from build123d import *

# Parameters (mm, degrees)
BOSS_EXTRUDE1_DEPTH          = 9
SKETCH2_R                    = 2.766798225
SKETCH2_W                    = 278
SKETCH2_H                    = 187
CUT_EXTRUDE1_DEPTH           = 2
SKETCH4_W                    = 10
SKETCH4_H                    = 4
CUT_EXTRUDE2_DEPTH           = 2
CUT_EXTRUDE2_DRAFT           = -19
CUT_EXTRUDE2_PROFILE_2_DEPTH = 2
CUT_EXTRUDE2_PROFILE_2_DRAFT = -19


with BuildPart() as part:
    # Sketch1 → Boss-Extrude1 (new body)
    with BuildSketch(Plane(origin=(0, 0, 0), x_dir=(1, 0, 0), z_dir=(0, 1, 0))):
        with BuildLine():
            Line((-177.6, 71.8), (90.4, 71.8))
            ThreePointArc((90.4, 71.8), (97.471067812, 68.871067812), (100.4, 61.8))
            Line((100.4, 61.8), (100.4, -127.2))
            ThreePointArc((100.4, -127.2), (97.471067812, -134.271067812), (90.4, -137.2))
            Line((90.4, -137.2), (-177.6, -137.2))
            ThreePointArc((-177.6, -137.2), (-184.671067812, -134.271067812), (-187.6, -127.2))
            Line((-187.6, -127.2), (-187.6, 61.8))
            ThreePointArc((-187.6, 61.8), (-184.671067812, 68.871067812), (-177.6, 71.8))
        make_face()
    extrude(amount=BOSS_EXTRUDE1_DEPTH)

    # Sketch2 → Cut-Extrude1 (cut)
    with BuildSketch(Plane(origin=(0, 9, 0), x_dir=(1, 0, 0), z_dir=(0, 1, 0))):
        with Locations(Location((-43.280764326, 66.757707022, 0), (0, 0, 270))):
            Circle(SKETCH2_R)
        with Locations((-43.280764326, -32.742292978)):
            Rectangle(SKETCH2_W, SKETCH2_H)
    extrude(amount=-CUT_EXTRUDE1_DEPTH, mode=Mode.SUBTRACT)


with BuildPart() as cut_extrude2_tool:
    # Sketch4 → Cut-Extrude2 (with draft: the straight prism first)
    with BuildSketch(Plane.ZY.offset(187.6)):
        with Locations((-11.8, 4.5)):
            Rectangle(SKETCH4_W, SKETCH4_H)
    extrude(amount=-CUT_EXTRUDE2_DEPTH)
    # Cut-Extrude2: the draft: its side faces are tilted about the plane it starts from
    cut_extrude2_sides = [cut_extrude2_tool.faces().sort_by_distance(p)[0] for p in [
        (-186.6, 6.5, -11.8),
        (-186.6, 4.5, -16.8),
        (-186.6, 2.5, -11.8),
        (-186.6, 4.5, -6.8),
    ]]
    draft(cut_extrude2_sides, Plane.ZY.offset(187.6), CUT_EXTRUDE2_DRAFT)


with BuildPart() as part_1:
    add(part.part)

    # Cut-Extrude2: cut by cut_extrude2_tool
    add(cut_extrude2_tool.part, mode=Mode.SUBTRACT)


with BuildPart() as cut_extrude2_profile_2_tool:
    # Sketch4 → Cut-Extrude2 profile 2 (with draft: the straight prism first)
    with BuildSketch(Plane.ZY.offset(187.6)):
        with Locations((18.2, 4.5)):
            Rectangle(SKETCH4_W, SKETCH4_H)
    extrude(amount=-CUT_EXTRUDE2_PROFILE_2_DEPTH)
    # Cut-Extrude2 profile 2: the draft: its side faces are tilted about the plane it starts from
    cut_extrude2_profile_2_sides = [cut_extrude2_profile_2_tool.faces().sort_by_distance(p)[0] for p in [
        (-186.6, 2.5, 18.2),
        (-186.6, 4.5, 23.2),
        (-186.6, 6.5, 18.2),
        (-186.6, 4.5, 13.2),
    ]]
    draft(cut_extrude2_profile_2_sides, Plane.ZY.offset(187.6), CUT_EXTRUDE2_PROFILE_2_DRAFT)


with BuildPart() as part_2:
    add(part_1.part)

    # Cut-Extrude2 profile 2: cut by cut_extrude2_profile_2_tool
    add(cut_extrude2_profile_2_tool.part, mode=Mode.SUBTRACT)


solid = part_2.part
Here's how the part is built. I have some questions about the finished solid (model axes, mm). A direction names the side the tool comes from. Round coordinates to 2 decimals unless told otherwise and drop trailing zeros. Write each loop counter-clockwise with the first axis right and the second up, starting at its lowest first coordinate (ties: lowest second). Pieces come first, ordered by that corner, then holes.
1. Will these pins go through, and if not, where does the flat tip stop? pin 1 Ø8 at (x, z) = (19.5, 106) entering from +Y; pin 2 Ø0.8 at (y, z) = (4, -13.5) entering from -X.
2. Suppose I cut it at B-B (x = -73.5). List the corners of the cut face in (y, z) for me, and give its area (3 significant figures).
3. I need wall thicknesses on L1, parallel to Z at x = 44.5, y = 8; L2, parallel to X at y = 8, z = 68; L3, parallel to Y at x = 14.5, z = 117. Which ranges of each line are inside material? Lowest first, please.
4. If we mould it in two halves opening along X, with no side actions, what happens to faces 1 (the flat face through (-187.6, 4, 34)), 2 (the flat face through (-45, 7, 31)), 3 (the cylindrical face through (-42.45, 8.01, -64.12)), 4 (the flat face through (-45, 4, -71.8))? For each: released by +X, released by -X, zero draft, split by the parting line, or undercut.
5. For faces 5 (the cylindrical face through (-184.75, 4.44, -68.79)), 6 (the flat face through (-43, 7, -67)), which set-ups out of +Z, -Z, +X, -X, +Y, -Y let a thin tool reach every point of the face, with its end or its side?
6. Suppose I cut it at A-A (z = 114). List the corners of the cut face in (x, y) for me.
Answer sheet:
1. pin 1: stops at y = 7
1. pin 2: stops at x = -185.6
2. outline: (0, -71.8) - (9, -71.8) - (9, -60.76) - (7, -60.76) - (7, 126.24) - (9, 126.24) - (9, 137.2) - (0, 137.2) - close
2. area: 1,510 mm2
3. L1: z = -71.8 to -60.76, 126.24 to 137.2
3. L2: x = -187.6 to -182.28, 95.72 to 100.4
3. L3: y = 0 to 7
4. face 1: released by -X
4. face 2: undercut
4. face 3: undercut
4. face 4: zero draft
5. face 5: -Z, -X, +Y, -Y
5. face 6: +Y
6. outline: (-187.6, 0) - (100.4, 0) - (100.4, 9) - (95.72, 9) - (95.72, 7) - (-182.28, 7) - (-182.28, 9) - (-187.6, 9) - close
